Geometry check sheet. Reference: the model listing, model coordinates, mm. Coordinates: 2 decimals unless noted, no trailing zeros. Loops run counter-clockwise (first coordinate to the right, second up) from the corner with the lowest first, then second, coordinate; pieces in that order, holes last. Notation, with made-up numbers: (23, -16) - (48, -16) arc R24 ccw to (48, 5) - close; hole circle Ø3 at (-1.5, -37.75). An arc over 180 degrees is marked (long way). One line per item, written item: value.
from build123d import *

# Parameters (mm, degrees)
BOSS_EXTRUDE1_DEPTH      = 1.5
BOSS_EXTRUDE1_DEPTH_BACK = 1.5
SKETCH3_W                = 152
SKETCH3_H                = 25
CUT_EXTRUDE1_DEPTH       = 520.533194562
SKETCH4_R                = 19.119387796
SKETCH4_R_2              = 47.191393473
SKETCH4_R_3              = 35.18699184
SKETCH4_R_4              = 12.586978738
SKETCH4_R_5              = 11.189603354
SKETCH4_R_6              = 21.557380713
SKETCH4_R_7              = 14.984143728
SKETCH4_R_8              = 11.239174992
SKETCH4_R_9              = 8.41496245
CUT_EXTRUDE2_DEPTH       = 10
FILLET1_R                = 3


with BuildPart() as part:
    # Sketch2 → Boss-Extrude1 (new, two sides)
    with BuildSketch(Plane(origin=(0, 0, 0), x_dir=(0, 0, -1), z_dir=(1, 0, 0))) as boss_extrude1_sk:
        Polygon((0, 67.22485033), (205.165503831, 48.288859026), (513.4, -0.530689138), (513.4, -22.650154351), (205.250409944, -63.717607751), (0, -79.537288439), (-70, -79.537288439), (-70, -69.537288439), (0, 17.22485033), align=None)
    extrude(amount=BOSS_EXTRUDE1_DEPTH)
    extrude(boss_extrude1_sk.sketch, amount=-BOSS_EXTRUDE1_DEPTH_BACK)

    # Sketch3 → Cut-Extrude1 (cut, through all)
    with BuildSketch(Plane(origin=(1.5, 0, 0), x_dir=(0, 0, -1), z_dir=(1, 0, 0))):
        with Locations((443.4, 17.5)):
            Rectangle(SKETCH3_W, SKETCH3_H)
    extrude(amount=-CUT_EXTRUDE1_DEPTH, mode=Mode.SUBTRACT)

    # Sketch4 → Cut-Extrude2 (cut)
    with BuildSketch(Plane(origin=(1.5, 0, 0), x_dir=(0, 0, -1), z_dir=(1, 0, 0))):
        with Locations((-22.865600385, -55.069339131)):
            Circle(SKETCH4_R)
        with Locations((55.752747866, -6.379566635)):
            Circle(SKETCH4_R_2)
        with Locations((268.826339435, -6.379566635)):
            Circle(SKETCH4_R_3)
        with Locations((225.050213704, 28.462655886)):
            Circle(SKETCH4_R_4)
        with Locations((17.336964062, 48.563938109)):
            Circle(SKETCH4_R_5)
        with Locations((225.050213704, -40.775093995)):
            Circle(SKETCH4_R_4)
        with Locations((327.790100624, -26.927544019)):
            Circle(SKETCH4_R_4)
        with Locations((327.790100624, 9.701459144)):
            Circle(SKETCH4_R_4)
        with Locations((149.867646424, 23.293890716)):
            Circle(SKETCH4_R_6)
        with Locations((149.867646424, -35.180680846)):
            Circle(SKETCH4_R_6)
        with Locations((379.3514003, -16.442535715)):
            Circle(SKETCH4_R_7)
        with Locations((425.129239545, -13.376077584)):
            Circle(SKETCH4_R_8)
        with Locations((465.431260698, -10.528652176)):
            Circle(SKETCH4_R_9)
    extrude(amount=-CUT_EXTRUDE2_DEPTH, mode=Mode.SUBTRACT)

    # Fillet1
    fillet1_edges = [part.edges().sort_by_distance(p)[0] for p in [
        (0, 22.593439149, -367.4),
        (0, 5, -367.4),
    ]]
    fillet(fillet1_edges, radius=FILLET1_R)


solid = part.part
(1) Cross-section at C-C on z = -218.5. Record the cut outline in (x, y).
Reply:
outline: (-1.5, -61.95) - (1.5, -61.95) - (1.5, -51.52) - (-1.5, -51.52) - close; (-1.5, -30.03) - (1.5, -30.03) - (1.5, 17.71) - (-1.5, 17.71) - close; (-1.5, 39.21) - (1.5, 39.21) - (1.5, 46.18) - (-1.5, 46.18) - close
(2) Cross-section at A-A on z = -49.5. Record the cut outline in (x, y), and give its area (3 significant figures).
Reply:
outline: (-1.5, -75.72) - (1.5, -75.72) - (1.5, -53.15) - (-1.5, -53.15) - close; (-1.5, 40.4) - (1.5, 40.4) - (1.5, 62.66) - (-1.5, 62.66) - close
area: 134 mm2
(3) Cross-section at B-B on x = -0.95. State how many separate pieces and enclosed holes the cut face has, and give its area (3 significant figures).
Reply:
separate pieces: 1
enclosed holes: 13
area: 31,300 mm2
(4) Material ranges on probe 1 along Z at (x, y) = (0.6, -7.5); probe 2 along Z at (x, y) = (0.6, 18); probe 3 along Z at (x, y) = (0.05, 11.5), recorded low to high. Write a range as from..to.
Reply:
probe 1: -513.4..-473.28, -457.58..-434.71, -415.55..-391.37, -367.33..-304, -233.66..-102.93, -8.57..19.95
probe 2: -367.4..-337.25, -318.33..-294.2, -243.45..-232.05, -218.05..-170.76, -128.97..-96.16, -15.35..0
probe 3: -367.4..-340.25, -315.33..-299.13, -238.52..-167.91, -131.82..-99.43, -12.08..4.62
(5) Cross-section at D-D on z = -450. Record the cut outline in (x, y), and give its area (3 significant figures).
Reply:
outline: (-1.5, -31.1) - (1.5, -31.1) - (1.5, 5) - (-1.5, 5) - close
area: 108 mm2
(6) Go/stop test with flat-tipped pins: pin 1 Ø0.9 at (x, y) = (-0.5, 50) entering from +Z; pin 2 Ø1.5 at (x, y) = (0.5, 19.5) entering from -Z; pin 3 Ø22.5 at (y, z) = (-40.78, -225.05) entering from +X. Record where each tip stops, or that it passes through.
Reply:
pin 1: z = 0
pin 2: z = -367.4
pin 3: through
